The model under review builds one solid part; all positions refer to its coordinate system, in mm. Round coordinates to 2 decimals unless told otherwise and drop trailing zeros. Loops run counter-clockwise (first coordinate to the right, second up) from the corner with the lowest first, then second, coordinate; pieces in that order, holes last. Notation, with made-up numbers: (58, 75.5) -> (63, 75.5) arc R23 cw to (63, 98.5) -> close; hole circle Ø2 at (65.25, 45.5). An arc over 180 degrees is marked (long way). Use a Markdown table: item, result. Add a question column.
1) Mouldability with a two-part tool opening along X and no side actions: class faces 1 (the flat face through (-1, -250, 6)), 2 (the cylindrical face through (-0.651, 195.043, 5.916)), 3 (the flat face through (-45, 3, 6)) as released by +X, released by -X, zero draft, split by the parting line, or undercut.
2) Insertion check: pin 1 (8 mm diameter, centred on x = 31.5, y = -136, fed in from -Z). The pin has a flat end and moves straight along its axis. Give the tip position at first contact, or say it passes through.
3) Wall thickness on probe 1 along Y at (x, z) = (0, 7); probe 2 along Y at (x, z) = (4.5, 8.25); probe 3 along X at (y, z) = (-31, 1.25): over which ranges is each line inside the solid? List them lowest first.
4) Consider section B-B on x = 0. Give the boundary of the cut face in (y, z).
5) Consider section A-A on y = -200. Give the boundary of the cut face in (x, z), plus the area to 3 significant figures.
Autodesk Inventor part; units mm, degrees
ref_plane "Work Plane1" through (0, 0, 0) normal (0, 0, 1) x (1, 0, 0)
ref_plane "YZ Plane" through (0, 0, 0) normal (1, 0, 0) x (0, 1, 0)
ref_plane "XZ Plane" through (0, 0, 0) normal (0, 1, 0) x (-1, 0, 0)
ref_plane "Work Plane1" through (0, 0, 0) normal (0, 0, 1) x (1, 0, 0)
sketch "Sketch1" plane through (0, 0, 0) normal (0, 0, 1) x (1, 0, 0)
  line L0 (-45, -250) -> (45, -250)
  line L1 (45, -250) -> (45, 250)
  line L2 (45, 250) -> (-45, 250)
  line L3 (-45, 250) -> (-45, -250)
  line L4 (0, -250) -> (0, 250) construction
  circle A0 centre (0, -200) radius 5
  line L5 (-45, 0) -> (126, 0) construction
  circle A1 centre (0, 200) radius 5
  dimension "d0" = 90
  dimension "d1" = 500
  dimension "d10" = 10
  dimension "d11" = 200
extrude "Extrusion1" add sketch "Sketch1" along normal blind 12
fillet "Fillet1" radius 2 4 edges at (-45, 0, 12) (-45, 0, 0) (45, 0, 12) (45, 0, 0)
properties part number "doga_short" material "Wood (Oak)"
Result set:
| question | item | result |
|---|---|---|
| 1 | face 1 | zero draft |
| 1 | face 2 | undercut |
| 1 | face 3 | released by -X |
| 2 | pin 1 | z = 0 |
| 3 | probe 1 | -250 to -205, -195 to 195, 205 to 250 |
| 3 | probe 2 | -250 to -202.18, -197.82 to 197.82, 202.18 to 250 |
| 3 | probe 3 | -44.85 to 44.85 |
| 4 | outline | (-250, 0) -> (-205, 0) -> (-205, 12) -> (-250, 12) -> close; (-195, 0) -> (195, 0) -> (195, 12) -> (-195, 12) -> close; (205, 0) -> (250, 0) -> (250, 12) -> (205, 12) -> close |
| 5 | outline | (-45, 2) arc R2 ccw to (-43, 0) -> (-5, 0) -> (-5, 12) -> (-43, 12) arc R2 ccw to (-45, 10) -> close; (5, 0) -> (43, 0) arc R2 ccw to (45, 2) -> (45, 10) arc R2 ccw to (43, 12) -> (5, 12) -> close |
| 5 | area | 957 mm2 |
